Could you check a few things on this model? Use its own coordinates, in mm. Coordinates: 2 decimals unless noted, no trailing zeros. Loops run counter-clockwise (first coordinate to the right, second up) from the corner with the lowest first, then second, coordinate; pieces in that order, holes last. Notation, with made-up numbers: (75, 63.5) - (105, 63.5) arc R28 cw to (105, 92.5) - close; hole circle Ø10 at (48.25, 34.5). An arc over 180 degrees is marked (long way). Use CSV: the item, a comma, the result in double quotes.
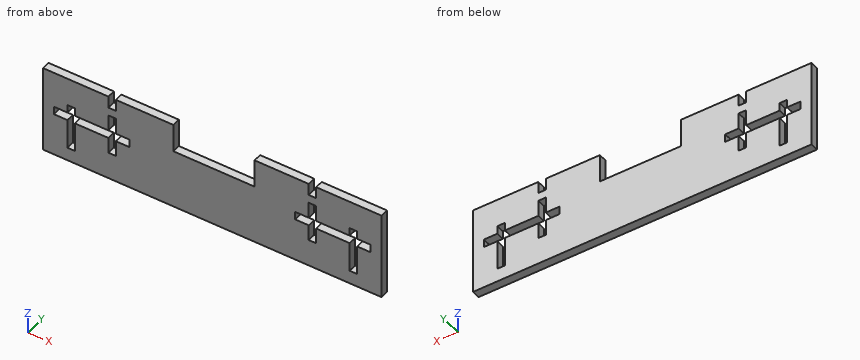
from build123d import *

# Parameters (mm, degrees)
SKETCH1_W           = 250
SKETCH1_H           = 65
BOSS_EXTRUDE1_DEPTH = 6
SKETCH2_W           = 5.5
SKETCH2_H           = 34
SKETCH2_H_2         = 47.5
CUT_EXTRUDE1_DEPTH  = 259.381500886
SKETCH3_W           = 60
SKETCH3_H           = 21
CUT_EXTRUDE2_DEPTH  = 259.381500886
SKETCH4_W           = 55.75
SKETCH4_H           = 6
CUT_EXTRUDE3_DEPTH  = 259.381500886
SKETCH5_W           = 5.5
SKETCH5_H           = 6.2
BOSS_EXTRUDE2_DEPTH = 6


with BuildPart() as part:
    # Sketch1 → Boss-Extrude1 (new body)
    with BuildSketch(Plane(origin=(0, 0, 0), x_dir=(1, 0, 0), z_dir=(0, 1, 0))):
        with Locations((125, 32.5)):
            Rectangle(SKETCH1_W, SKETCH1_H)
    extrude(amount=BOSS_EXTRUDE1_DEPTH)

    # Sketch2 → Cut-Extrude1 (cut, through all)
    with BuildSketch(Plane(origin=(0, 6, 0), x_dir=(1, 0, 0), z_dir=(0, 1, 0))):
        with Locations((20.75, 38)):
            Rectangle(SKETCH2_W, SKETCH2_H)
        with Locations((51, 21)):
            Rectangle(SKETCH2_W, SKETCH2_H_2)
        with Locations((199, 21)):
            Rectangle(SKETCH2_W, SKETCH2_H_2)
        with Locations((229.25, 38)):
            Rectangle(SKETCH2_W, SKETCH2_H)
    extrude(amount=-CUT_EXTRUDE1_DEPTH, mode=Mode.SUBTRACT)

    # Sketch3 → Cut-Extrude2 (cut, through all)
    with BuildSketch(Plane(origin=(0, 6, 0), x_dir=(1, 0, 0), z_dir=(0, 1, 0))):
        with Locations((126.25, 10.5)):
            Rectangle(SKETCH3_W, SKETCH3_H)
    extrude(amount=-CUT_EXTRUDE2_DEPTH, mode=Mode.SUBTRACT)

    # Sketch4 → Cut-Extrude3 (cut, through all)
    with BuildSketch(Plane(origin=(0, 6, 0), x_dir=(1, 0, 0), z_dir=(0, 1, 0))):
        with Locations((35.875, 30)):
            Rectangle(SKETCH4_W, SKETCH4_H)
    cut_extrude3 = extrude(amount=-CUT_EXTRUDE3_DEPTH, mode=Mode.SUBTRACT)

    # Sketch5 → Boss-Extrude2 (add)
    with BuildSketch(Plane(origin=(0, 6, 0), x_dir=(1, 0, 0), z_dir=(0, 1, 0))):
        with Locations((51, 11.9)):
            Rectangle(SKETCH5_W, SKETCH5_H)
    boss_extrude2 = extrude(amount=-BOSS_EXTRUDE2_DEPTH)

    # Mirror1: Cut-Extrude3, Boss-Extrude2 across plane
    add(cut_extrude3.mirror(Plane(origin=(125, 0, 0), x_dir=(0, 0, 1), z_dir=(1, 0, 0))), mode=Mode.SUBTRACT)
    add(boss_extrude2.mirror(Plane(origin=(125, 0, 0), x_dir=(0, 0, 1), z_dir=(1, 0, 0))))


solid = part.part
(1) Suppose I cut it at D-D (y = 3.2). State how many separate pieces and enclosed holes the cut face has, plus the area to 3 significant figures.
Computed:
separate pieces,"1"
enclosed holes,"2"
area,"13,700 mm²"
(2) Suppose I cut it at A-A (z = -36). Write out the boundary of the cut face in (x, y).
Computed:
outline,"(0, 0) - (18, 0) - (18, 6) - (0, 6) - close; (23.5, 0) - (48.25, 0) - (48.25, 6) - (23.5, 6) - close; (53.75, 0) - (196.25, 0) - (196.25, 6) - (53.75, 6) - close; (201.75, 0) - (226.5, 0) - (226.5, 6) - (201.75, 6) - close; (232, 0) - (250, 0) - (250, 6) - (232, 6) - close"
(3) Please list where these lines run through material, in increasing order: line 1 (X direction, y = 2, z = -18.5); line 2 (X direction, y = 5.15, z = -52); line 3 (X direction, y = 4.55, z = -38.5).
Computed:
line 1,"x = 0 to 48.25, 53.75 to 96.25, 156.25 to 196.25, 201.75 to 250"
line 2,"x = 0 to 18, 23.5 to 226.5, 232 to 250"
line 3,"x = 0 to 18, 23.5 to 48.25, 53.75 to 196.25, 201.75 to 226.5, 232 to 250"
(4) Will this pin go through, and if not, where does the flat tip stop? pin 1 (1.6 mm diameter, centred on x = 52, y = 4, fed in from +Z).
Computed:
pin 1,"stops at z = -8.8"
(5) Suppose I cut it at B-B (z = -49). Write out the boundary of the cut face in (x, y).
Computed:
outline,"(0, 0) - (18, 0) - (18, 6) - (0, 6) - close; (23.5, 0) - (226.5, 0) - (226.5, 6) - (23.5, 6) - close; (232, 0) - (250, 0) - (250, 6) - (232, 6) - close"
(6) Suppose I cut it at C-C (x = 39). Write out the boundary of the cut face in (y, z), plus the area to 3 significant figures.
Computed:
outline,"(0, -65) - (6, -65) - (6, -33) - (0, -33) - close; (0, -27) - (6, -27) - (6, 0) - (0, 0) - close"
area,"354 mm²"
